Autodesk Inventor part; units mm, degrees
ref_plane "YZ Plane" through (0, 0, 0) normal (1, 0, 0) x (0, 1, 0)
ref_plane "XZ Plane" through (0, 0, 0) normal (0, 1, 0) x (-1, 0, 0)
ref_plane "XY Plane" through (0, 0, 0) normal (0, 0, 1) x (1, 0, 0)
sketch "Sketch1" plane through (0, 0, 0) normal (0, 0, 1) x (1, 0, 0)
  line L0 (0, 0) -> (152.4, 0)
  line L1 (152.4, 0) -> (152.4, -25.4)
  line L2 (152.4, -25.4) -> (0, -25.4)
  line L3 (0, -25.4) -> (0, 0)
  dimension "d0" = 152.4
  dimension "d1" = 25.4
extrude "Extrusion1" add sketch "Sketch1" along normal blind 6.35
sketch "Sketch4" plane through (0, 0, 6.35) normal (0, 0, 1) x (1, 0, 0)
  circle A0 centre (63.5, -2.921) radius 1.3589
  circle A1 centre (56.5852, -5.7852) radius 1.3589
  circle A2 centre (53.721, -12.7) radius 1.3589
  circle A3 centre (56.5852, -19.6148) radius 1.3589
  circle A4 centre (63.5, -22.479) radius 1.3589
  circle A5 centre (70.4148, -19.6148) radius 1.3589
  circle A6 centre (73.279, -12.7) radius 1.3589
  circle A7 centre (70.4148, -5.7852) radius 1.3589
  line L0 (0, -25.4) -> (152.4, -25.4)
  line L1 (152.4, 0) -> (0, 0)
  line L2 (152.4, -25.4) -> (152.4, 0)
  point P0 (9.525, 0)
  point P1 (63.5, -12.7)
  point P2 (254, 0)
  point P3 (254, -19.05)
  point P4 (63.5, -12.7)
  point P5 (63.5, -12.7)
  point P6 (63.5, -12.7)
  point P7 (63.5, -12.7)
  point P8 (63.5, -12.7)
  point P9 (63.5, -12.7)
  point P10 (63.5, -12.7)
  point P11 (11.43, 0)
  dimension "d71" = 2.7178
  dimension "d72" = 9.779
  dimension "d73" = 0
  dimension "d76" = 360
  dimension "d85" = 25.4
  dimension "d86" = 12.7
  dimension "d87" = 88.9
sketch "Sketch9" plane through (152.4, -25.4, 0) normal (0, -1, 0) x (1, 0, 0)
  line L0 (0, 0) -> (0, 6.35)
  line L1 (0, 0) -> (43.9941, 25.4)
  line L2 (0, 0) -> (50.8, 0) construction
  line L3 (0, 6.35) -> (43.9941, 31.75)
  line L4 (0, 6.35) -> (50.8, 6.35) construction
  line L5 (43.9941, 31.75) -> (43.9941, 25.4)
  point P0 (-152.4, 0)
  dimension "d53" = 50.8
  dimension "d54" = 30
  dimension "d55" = 50.8
  dimension "d56" = 30
extrude "Extrusion9" add sketch "Sketch9" against normal up to surface (25.4 mm away)
sketch "Sketch10" plane through (196.3941, -25.4, 25.4) normal (0.5, 0, -0.866) x (-0.866, 0, -0.5)
  line L0 (0, 0) -> (50.8, 0)
  line L1 (50.8, 25.4) -> (0, 25.4)
  line L2 (0, 0) -> (0, 25.4)
  circle A0 centre (38.1, 12.7) radius 2.3368
  circle A1 centre (25.4, 12.7) radius 2.3368
  circle A2 centre (12.7, 12.7) radius 6.35
  point P0 (182.7823, 25.4)
  dimension "d59" = 25.4
  dimension "d60" = 12.7
  dimension "d61" = 12.7
  dimension "d62" = 12.7
  dimension "d63" = 12.7
  dimension "d64" = 25.4
  dimension "d65" = 38.1
  dimension "d66" = 4.6736
  dimension "d67" = 4.6736
  dimension "d68" = 12.7
extrude "Extrusion10" cut sketch "Sketch10" against normal through all
hole "Hole1" at (70.4148, -5.7852, 6.35) at (73.279, -12.7, 6.35) at (70.4148, -19.6148, 6.35) at (63.5, -22.479, 6.35) at (56.5852, -19.6148, 6.35) at (53.721, -12.7, 6.35) at (56.5852, -5.7852, 6.35) at (63.5, -2.921, 6.35) direction (0, 0, -1) diameter 2.7178 end through all
equation "\"d55\" = d53"
properties part number "Wheel Arms"
Model file for the job. Use its own axes, mm. A direction names the side the tool comes from. Give positions to 0.01 mm unless a question says otherwise; leave off trailing zeros. Loops run counter-clockwise (first coordinate to the right, second up) from the corner with the lowest first, then second, coordinate; pieces in that order, holes last.
1) Flat gauge pins, fed straight in: pin 1 Ø1.6 at (x, y) = (63.5, -22.479) entering from +Z; pin 2 Ø12.5 at (x, y) = (93, -10) entering from +Z; pin 3 Ø12 at (y, z) = (-14, 7) entering from +X; pin 4 Ø10 at (y, z) = (-16.5, 19) entering from +X. Where does each tip first touch, or does it go through?
2) Tool access for faces 1 (the flat face through (75, -13, 6.35)), 2 (the cylindrical face through (181.5, -18.33, 19.93)): list every direction of +Z, -Z, +X, -X, +Y, -Y with a clear straight run to the whole face (end or side of a thin tool).
3) Pull direction Y, two halves, no side cores. Call faces 3 (the cylindrical face through (174.647, -14.122, 15.975)), 4 (the flat face through (0, -13, 3)), 5 (the flat face through (99, -25.4, 4)): +Y half, -Y half, draft (parallel to the pull), parting line (faces both ways), or undercut.
4) Saw through at A-A (x = 106). Write the cut outline in (y, z).
5) Wall check: line 1 (Y direction, x = 63.5, z = 3); line 2 (Z direction, x = 16.5, y = -11); line 3 (X direction, y = -12.5, z = 3.5). Give the ranges that are in metal, low to high.
Answer block:
1. pin 1: passes through
1. pin 2: stops at z = 6.35
1. pin 3: stops at x = 174.77
1. pin 4: stops at x = 193.97
2. face 1: +Z, -X, +Y, -Y
2. face 2: none
3. face 3: undercut
3. face 4: draft
3. face 5: -Y half
4. outline: (-25.4, 0) - (0, 0) - (0, 6.35) - (-25.4, 6.35) - close
5. line 1: y = -25.4 to -23.84, -21.12 to -4.28, -1.56 to 0
5. line 2: z = 0 to 6.35
5. line 3: x = 0 to 52.38, 55.07 to 71.93, 74.62 to 158.46
